```python
from build123d import *

# Parameters (mm, degrees)
BOSS_EXTRUDE2_DEPTH = 1
SKETCH2_R           = 1
BOSS_EXTRUDE3_DEPTH = 8


with BuildPart() as part:
    # Sketch1 → Boss-Extrude2 (new body)
    with BuildSketch(Plane.XY):
        with BuildLine():
            Line((-0.5, -1.5), (0.5, -1.5))
            ThreePointArc((0.5, -1.5), (1.207106781, -1.207106781), (1.5, -0.5))
            Line((1.5, -0.5), (1.5, 0.5))
            ThreePointArc((1.5, 0.5), (1.207106781, 1.207106781), (0.5, 1.5))
            Line((0.5, 1.5), (-0.5, 1.5))
            ThreePointArc((-0.5, 1.5), (-1.207106781, 1.207106781), (-1.5, 0.5))
            Line((-1.5, 0.5), (-1.5, -0.5))
            ThreePointArc((-1.5, -0.5), (-1.207106781, -1.207106781), (-0.5, -1.5))
        make_face()
    extrude(amount=BOSS_EXTRUDE2_DEPTH)

    # Sketch2 → Boss-Extrude3 (add)
    with BuildSketch(Plane.XY.offset(1)):
        Circle(SKETCH2_R)
    extrude(amount=BOSS_EXTRUDE3_DEPTH)


solid = part.part
```
Input: part model. Units: mm. Frame: model coordinates. A direction names the side the tool comes from. Round coordinates to 2 decimals unless told otherwise and drop trailing zeros. Loops run counter-clockwise (first coordinate to the right, second up) from the corner with the lowest first, then second, coordinate; pieces in that order, holes last. Notation, with made-up numbers: M -13.75,56.5 L 14.25,56.5 A20 cw 14.25,73.5 Z; hole C 41.5,3 d4. An arc over 180 degrees is marked long. Answer in a Markdown table with one row per item. Add a question column.
1. Ray query, probe 1 along Z at (x, y) = (0.85, 1.35); probe 2 along X at (y, z) = (0.6, 8.75); probe 3 along X at (y, z) = (-0.9, 1.75). Return the intervals inside material, ascending.
2. Section A-A (y = 0). Output: boundary loops of the cut face in (x, z).
3. Section C-C (z = 4.25). Output: boundary loops of the cut face in (x, y), and give its area (3 significant figures).
4. Contact query for a flat-ended pin moving along its axis: pin 1 (1 mm diameter, centred on x = -0.5, z = 5, fed in from -Y). Output: stop coordinate, or through.
5. Set-up query: faces 1 (the face through (0, -1, 5)), 2 (the face through (-1.5, 0, 0.5)). Return all of +Z, -Z, +X, -X, +Y, -Y with unobstructed straight access to the full face (end or side cutting, diameter ignored); none if empty.
Values follow:
| question | item | result |
|---|---|---|
| 1 | probe 1 | 0 to 1 |
| 1 | probe 2 | -0.8 to 0.8 |
| 1 | probe 3 | -0.44 to 0.44 |
| 2 | outline | M -1.5,0 L 1.5,0 L 1.5,1 L 1,1 L 1,9 L -1,9 L -1,1 L -1.5,1 Z |
| 3 | outline | C 0,0 d2 |
| 3 | area | 3.14 mm^2 |
| 4 | pin 1 | y = -1 |
| 5 | face 1 | +Z |
| 5 | face 2 | +Z, -Z, -X, +Y, -Y |
